```python
from build123d import *

# Parameters (mm, degrees)
SKETCH1_W              = 40
SKETCH1_H              = 35.362964007
BOSS_EXTRUDE1_DEPTH    = 50
SKETCH2_W              = 35.362964007
SKETCH2_H              = 5.5
BOSS_EXTRUDE2_DEPTH    = 22
SKETCH3_R              = 2.5
SKETCH3_R_2            = 1
SKETCH3_R_3            = 1.025
BOSS_EXTRUDE3_DEPTH    = 14
D_GAGEMENT_M71_D       = 8
BOSS_EXTRUDE4_DEPTH    = 35.362964
SKETCH8_W              = 12.572018863
SKETCH8_H              = 35.362964007
BOSS_EXTRUDE5_DEPTH    = 15.144107649
D_GAGEMENT_M2_53_D     = 3.1
D_GAGEMENT_M2_53_DEPTH = 6
D_GAGEMENT_M2_53_TIP   = 0.931333959
D_GAGEMENT_M2_51_D     = 3.1
D_GAGEMENT_M2_51_DEPTH = 6
D_GAGEMENT_M2_51_TIP   = 0.931333959


with BuildPart() as part:
    # Sketch1 → Boss-Extrude1 (new body)
    with BuildSketch(Plane(origin=(0, 0, 0), x_dir=(1, 0, 0), z_dir=(0, 1, 0))):
        with Locations((7.230679314, -2.945715381)):
            Rectangle(SKETCH1_W, SKETCH1_H)
    extrude(amount=BOSS_EXTRUDE1_DEPTH)

    # Sketch2 → Boss-Extrude2 (add)
    with BuildSketch(Plane.ZY.offset(12.769320686)):
        with Locations((2.945715381, 2.75)):
            Rectangle(SKETCH2_W, SKETCH2_H)
    extrude(amount=BOSS_EXTRUDE2_DEPTH)

    # Sketch3 → Boss-Extrude3 (add)
    # profile 1 of 4: a face of its own
    with BuildSketch(Plane(origin=(0, 50, 0), x_dir=(1, 0, 0), z_dir=(0, 1, 0))):
        with Locations(Location((3.355679314, -3.889233377, 0), (0, 0, 90))):
            Circle(SKETCH3_R)
        with Locations(Location((3.355679314, -3.889233377, 0), (0, 0, 270))):
            Circle(SKETCH3_R_2, mode=Mode.SUBTRACT)
    # profile 2 of 4: a face of its own
    with BuildSketch(Plane(origin=(0, 50, 0), x_dir=(1, 0, 0), z_dir=(0, 1, 0))):
        with Locations(Location((24.355679314, -3.764233372, 0), (0, 0, 90))):
            Circle(SKETCH3_R)
        with Locations(Location((24.355679314, -3.764233372, 0), (0, 0, 270))):
            Circle(SKETCH3_R_3, mode=Mode.SUBTRACT)
    # profile 3 of 4: a face of its own
    with BuildSketch(Plane(origin=(0, 50, 0), x_dir=(1, 0, 0), z_dir=(0, 1, 0))):
        with Locations(Location((3.355679314, 8.610766623, 0), (0, 0, 90))):
            Circle(SKETCH3_R)
        with Locations(Location((3.355679314, 8.610766623, 0), (0, 0, 270))):
            Circle(SKETCH3_R_3, mode=Mode.SUBTRACT)
    # profile 4 of 4: a face of its own
    with BuildSketch(Plane(origin=(0, 50, 0), x_dir=(1, 0, 0), z_dir=(0, 1, 0))):
        with Locations(Location((24.355307287, 8.735766623, 0), (0, 0, 90))):
            Circle(SKETCH3_R)
        with Locations(Location((24.355307287, 8.735766623, 0), (0, 0, 270))):
            Circle(SKETCH3_R_3, mode=Mode.SUBTRACT)
    extrude(amount=BOSS_EXTRUDE3_DEPTH)

    # Dégagement M71 (through all)
    with Locations(Plane(origin=(0, 0, 0), x_dir=(-1, 0, 0), z_dir=(0, -1, 0))):
        with Locations((24.769320686, -2.945715381)):
            Hole(D_GAGEMENT_M71_D / 2)

    # Sketch7 → Boss-Extrude4 (add)
    with BuildSketch(Plane.XY.offset(20.627197384)):
        Polygon((27.230679314, 34.010518151), (40.568594836, 65.144107649), (30.139889808, 65.144107649), (27.230679314, 50), align=None)
    extrude(amount=-BOSS_EXTRUDE4_DEPTH)

    # Sketch8 → Boss-Extrude5 (add)
    with BuildSketch(Plane(origin=(0, 50, 0), x_dir=(1, 0, 0), z_dir=(0, 1, 0))):
        with Locations((-6.483311255, -2.945715381)):
            Rectangle(SKETCH8_W, SKETCH8_H)
    extrude(amount=BOSS_EXTRUDE5_DEPTH)

    # Dégagement M2.53
    with Locations(Plane(origin=(0, 65.144107649, 0), x_dir=(1, 0, 0), z_dir=(0, 1, 0))):
        with Locations((-8.745252094, -3.961262734), (36.054747906, -3.961262734)):
            Hole(D_GAGEMENT_M2_53_D / 2, depth=D_GAGEMENT_M2_53_DEPTH)
            with Locations((0, 0, -(D_GAGEMENT_M2_53_DEPTH + D_GAGEMENT_M2_53_TIP / 2))):  # 118° drill point
                Cone(0, D_GAGEMENT_M2_53_D / 2, D_GAGEMENT_M2_53_TIP, mode=Mode.SUBTRACT)

    # Dégagement M2.51
    with Locations(Plane(origin=(0, 0, 0), x_dir=(-1, 0, 0), z_dir=(0, -1, 0))):
        with Locations((8.473719715, -2.945715381), (-20.230679314, -2.945715381)):
            Hole(D_GAGEMENT_M2_51_D / 2, depth=D_GAGEMENT_M2_51_DEPTH)
            with Locations((0, 0, -(D_GAGEMENT_M2_51_DEPTH + D_GAGEMENT_M2_51_TIP / 2))):  # 118° drill point
                Cone(0, D_GAGEMENT_M2_51_D / 2, D_GAGEMENT_M2_51_TIP, mode=Mode.SUBTRACT)


solid = part.part
```
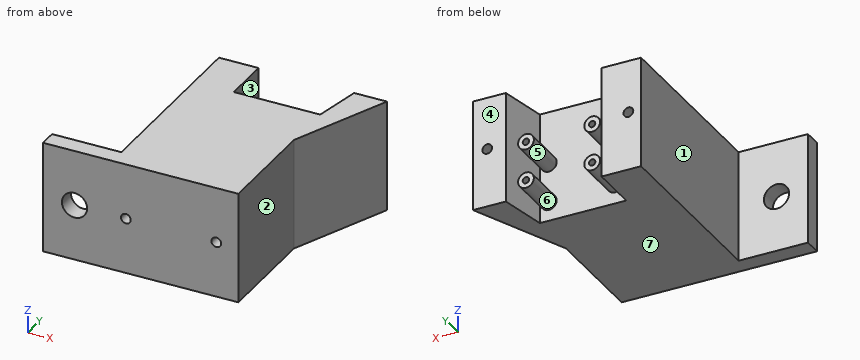
Model file for the job. Use its own axes, mm. Face numbers are marked on the shaded views. A direction names the side the tool comes from. Give positions to 0.01 mm unless a question says otherwise; leave off trailing zeros. Write each loop counter-clockwise with the first axis right and the second up, starting at its lowest first coordinate (ties: lowest second). Pieces come first, ordered by that corner, then holes. Notation, with made-up numbers: M 69,16 L 128,16 A26 cw 128,54 Z; hole C -23,-16 d3. An arc over 180 degrees is marked long. Use a Markdown table: item, result.
1) Pin check, flat tips, straight feed: pin 1 (2.5 mm diameter, centred on x = 36.05, z = 3.96, fed in from +Y); pin 2 (1.5 mm diameter, centred on y = 42, z = 13, fed in from -X); pin 3 (2.5 mm diameter, centred on x = 24.5, z = -8, fed in from +Y); pin 4 (10 mm diameter, centred on x = -21, y = 34, fed in from -Z). Stop position of each tip, or through.
Responses:
| item | result |
|---|---|
| pin 1 | stops at y = 58.97 |
| pin 2 | stops at x = -12.77 |
| pin 3 | stops at y = 64 |
| pin 4 | passes through |
2) Cut at C-C (x = -16.5). List the corners of the cut face in (y, z).
Responses:
| item | result |
|---|---|
| outline | M 0,-14.74 L 5.5,-14.74 L 5.5,20.63 L 0,20.63 Z |
3) Drill centre lines: line 1 (Y direction, x = -18, z = 3.5); line 2 (Y direction, x = 15, z = -4); line 3 (X direction, y = 27, z = 14). Where is each one in solid material? Low to high. Write a range as from..to.
Responses:
| item | result |
|---|---|
| line 1 | y = 0..5.5 |
| line 2 | y = 0..50 |
| line 3 | x = -12.77..27.23 |
4) Cut at B-B (y = 15.5). List the corners of the cut face in (x, z), and give its area (3 significant figures).
Responses:
| item | result |
|---|---|
| outline | M -12.77,-14.74 L 27.23,-14.74 L 27.23,20.63 L -12.77,20.63 Z |
| area | 1,410 mm2 |
5) Cut at A-A (z = 14). List the corners of the cut face in (x, y), and give its area (3 significant figures).
Responses:
| item | result |
|---|---|
| outline | M -34.77,0 L 27.23,0 L 27.23,34.01 L 40.57,65.14 L 30.14,65.14 L 27.23,50 L -0.2,50 L -0.2,65.14 L -12.77,65.14 L -12.77,5.5 L -34.77,5.5 Z |
| area | 2,500 mm2 |
6) Pull direction Z, two halves, no side cores. Call the marked faces 4, 5, 6 and 7: +Z half, -Z half, draft (parallel to the pull), parting line (faces both ways), or undercut.
Responses:
| item | result |
|---|---|
| face 4 | draft |
| face 5 | undercut |
| face 6 | undercut |
| face 7 | -Z half |
7) Tool access for the marked faces 1, 2 and 3: list every direction of +Z, -Z, +X, -X, +Y, -Y with a clear straight run to the whole face (end or side of a thin tool).
Responses:
| item | result |
|---|---|
| face 1 | +Z, -Z, -X, +Y |
| face 2 | +Z, -Z, +X, -Y |
| face 3 | +Z, -Z, +Y |
